Part print with two shaded views. Sizes in mm from the minimum x, y, z corner. Round coordinates to 2 decimals unless told otherwise and drop trailing zeros. Write each loop counter-clockwise with the first axis right and the second up, starting at its lowest first coordinate (ties: lowest second). Pieces come first, ordered by that corner, then holes. Notation, with made-up numbers: (40, 31.5) - (98, 31.5) arc R23 ccw to (98, 65.5) - close; hole circle Ø6 at (6, 38.5). An arc over 180 degrees is marked (long way). Answer as a JSON object with one key per item and string values. Group by question number.
Item 1: Slice it at A-A, the plane z = 4. List the corners of the cut face in (x, y), then the cut area to 3 significant figures.
Item 2: Slice it at D-D, the plane z = 1.25. List the corners of the cut face in (x, y).
Item 3: Flat gauge pin, fed straight in: pin 1 (3.5 mm diameter, centred on x = 4.54, z = 4, fed in from -Y). Where does the tip first touch, or does it go through?
Item 4: Two-plate mould, pull along Z, no slides. Class the marked faces 1, 2 and 3: +Z half, -Z half, draft (parallel to the pull), parting line (faces both ways), or undercut.
Item 5: Slice it at C-C, the plane x = 4. List the corners of the cut face in (y, z) (1 decimal).
Item 6: Probe line 1 (Z direction, x = 5, y = 2.45); line 2 (X direction, y = 1, z = 2.5) (1 decimal); line 3 (X direction, y = 2.4, z = 5.25) (1 decimal). List the from-to ranges inside material, lowest first. Write a range as from..to.
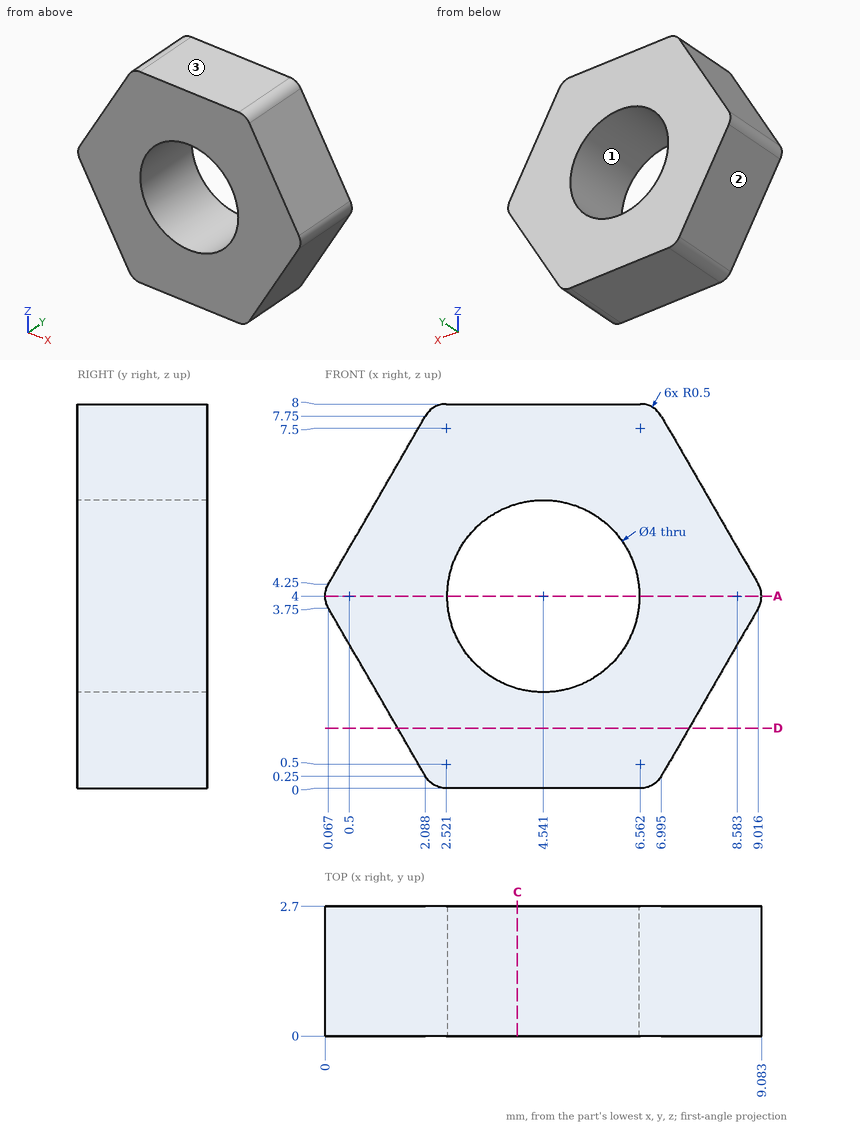
Geometry says:
{
 "1": {"outline": "(0, 0) - (2.54, 0) - (2.54, 2.7) - (0, 2.7) - close; (6.54, 0) - (9.08, 0) - (9.08, 2.7) - (6.54, 2.7) - close", "area": "13.7 mm^2"},
 "2": {"outline": "(1.51, 0) - (7.57, 0) - (7.57, 2.7) - (1.51, 2.7) - close"},
 "3": {"pin 1": "passes through"},
 "4": {"face 1": "undercut", "face 2": "-Z half", "face 3": "+Z half"},
 "5": {"outline": "(0, 0) - (2.7, 0) - (2.7, 2.1) - (0, 2.1) - close; (0, 5.9) - (2.7, 5.9) - (2.7, 8) - (0, 8) - close"},
 "6": {"line 1": "z = 0..2.05, 5.95..8", "line 2": "x = 0.8..3.2, 5.9..8.3", "line 3": "x = 0.6..3, 6.1..8.4"}
}
